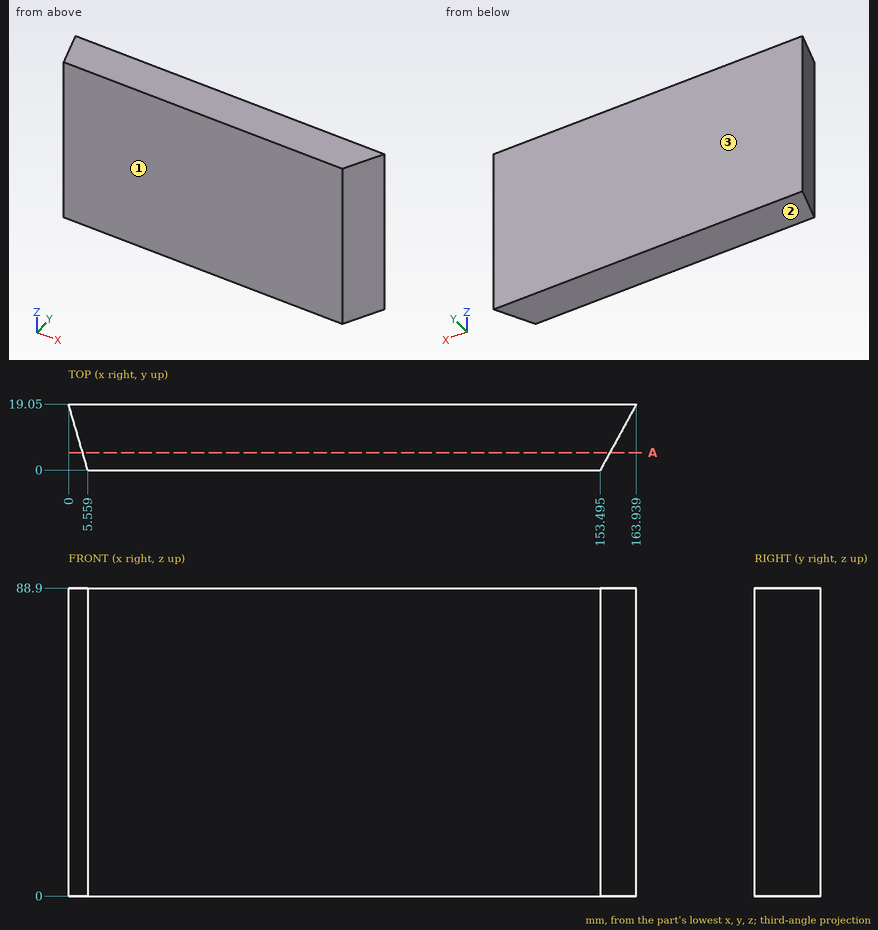
The figure shows three views and two pictorial views of one solid part (mm, origin at its lowest corner). Answer the questions. Give positions to 0.01 mm unless a question says otherwise; leave off trailing zeros. Write each loop counter-clockwise with the first axis right and the second up, starting at its lowest first coordinate (ties: lowest second). Pieces come first, ordered by that corner, then holes. Notation, with made-up numbers: (52, 56) - (99, 56) arc R13 cw to (99, 71) - close; hole circle Ø4 at (59, 66.5). An arc over 180 degrees is marked (long way). Use one line per item in the form item = value.
1. A cutting plane is placed at A-A (y = 5). Write down the section's boundary in (x, z).
Filled in:
outline = (4.1, 0) - (156.24, 0) - (156.24, 88.9) - (4.1, 88.9) - close
2. Each of these flat-tipped pins is pushed along its axis until it touches: pin 1 Ø4 at (y, z) = (12.5, 14.5) entering from +X (1 decimal); pin 2 Ø3 at (y, z) = (9, 40) entering from +X; pin 3 Ø8 at (x, y) = (59, 8) entering from -Z; pin 4 Ø1.5 at (y, z) = (9.5, 13) entering from -X. Where does it stop, or does it pass through?
Filled in:
pin_1 = 161.4
pin_2 = 159.25
pin_3 = 0
pin_4 = 2.57
3. Consider L1, parallel to X at y = 1, z = 37.5; L2, parallel to X at y = 9.25, z = 77 (1 decimal). Determine where each line is inside the solid, lowest interval first.
Filled in:
L1 = 5.27 to 154.04
L2 = 2.9 to 158.6
4. Determine the mould class of the marked faces 1, 2 and 3 for opening direction Y: released by +Y, released by -Y, zero draft, split by the parting line, or undercut.
Filled in:
face_1 = released by -Y
face_2 = zero draft
face_3 = released by +Y
